Read the model definition and answer for the solid it produces. Units are mm, in the model's axes. Coordinates: 2 decimals unless noted, no trailing zeros. Write each loop counter-clockwise with the first axis right and the second up, starting at its lowest first coordinate (ties: lowest second). Pieces come first, ordered by that corner, then holes.
Item 1: Section C-C (z = -12) is taken. Give the vertices of the cut face in (x, y).
Item 2: Straight lines are drawn through the part: probe 1 along Z at (x, y) = (36, 1.5); probe 2 along X at (y, z) = (0.35, -63.94); probe 3 along X at (y, z) = (1.05, -17). For each, find the intervals that lie inside material, in ascending order.
Item 3: Section B-B (x = 6) is taken. Give the vertices of the cut face in (y, z).
Item 4: Section A-A (z = -48) is taken. Give the vertices of the cut face in (x, y).
Item 5: Each of these flat-tipped pins is pushed along its axis until it touches: P1, Ø2, axis at y = 1.5, z = -30.5, coming from the -X side; P2, Ø1.2, axis at y = -0.5, z = -38, coming from the +X side. Where does it stop, or does it pass through?
from build123d import *

# Parameters (mm, degrees)
SKETCH5_W           = 36.75
SKETCH5_H           = 66.29
BOSS_EXTRUDE3_DEPTH = 1
FILLET1_R           = 2
FILLET2_R           = 2
SKETCH7_R           = 1
CUT_EXTRUDE1_DEPTH  = 2
SKETCH9_W           = 4.683907435
SKETCH9_H           = 11.166934783
SKETCH9_W_2         = 3.743745131
SKETCH9_H_2         = 8.450578132
SKETCH9_W_3         = 2.561846092
SKETCH9_H_3         = 4.440718541
SKETCH9_H_4         = 4.716987875
SKETCH9_W_4         = 5.346352719
SKETCH9_H_5         = 7.570803243
BOSS_EXTRUDE5_DEPTH = 3
SKETCH11_W          = 2
SKETCH11_H          = 1.271998182
SKETCH11_H_2        = 1.351132692
BOSS_EXTRUDE6_DEPTH = 1
SKETCH12_W          = 2
SKETCH12_H          = 2
BOSS_EXTRUDE7_DEPTH = 2
SKETCH13_W          = 29.25
SKETCH13_H          = 59.29
BOSS_EXTRUDE8_DEPTH = 1.5


with BuildPart() as part:
    # Sketch5 → Boss-Extrude3 (new body)
    with BuildSketch(Plane(origin=(0, 0, 0), x_dir=(1, 0, 0), z_dir=(0, 1, 0))):
        with Locations((18.375, 33.145)):
            Rectangle(SKETCH5_W, SKETCH5_H)
    extrude(amount=BOSS_EXTRUDE3_DEPTH)

    # Fillet1
    fillet1_edges = [part.edges().sort_by_distance(p)[0] for p in [
        (0, 0.5, 0),
    ]]
    fillet(fillet1_edges, radius=FILLET1_R)

    # Fillet2
    fillet2_edges = [part.edges().sort_by_distance(p)[0] for p in [
        (0, 0.5, -66.29),
        (36.75, 0.5, -66.29),
        (36.75, 0.5, 0),
    ]]
    fillet(fillet2_edges, radius=FILLET2_R)

    # Sketch7 → Cut-Extrude1 (cut)
    with BuildSketch(Plane(origin=(0, 1, 0), x_dir=(1, 0, 0), z_dir=(0, 1, 0))):
        with Locations(Location((2.15, 63.94, 0), (0, 0, 270))):
            Circle(SKETCH7_R)
        with Locations(Location((34.5, 63.94, 0), (0, 0, 270))):
            Circle(SKETCH7_R)
        with Locations(Location((2.15, 2.52, 0), (0, 0, 270))):
            Circle(SKETCH7_R)
        with Locations(Location((34.5, 2.52, 0), (0, 0, 270))):
            Circle(SKETCH7_R)
    extrude(amount=-CUT_EXTRUDE1_DEPTH, mode=Mode.SUBTRACT)

    # Sketch9 → Boss-Extrude5 (add)
    with BuildSketch(Plane(origin=(0, 1, 0), x_dir=(1, 0, 0), z_dir=(0, 1, 0))):
        with Locations((2.341953718, 11.952713426)):
            Rectangle(SKETCH9_W, SKETCH9_H)
        with Locations((34.878127435, 23.466626346)):
            Rectangle(SKETCH9_W_2, SKETCH9_H_2)
        with Locations((35.469076954, 15.315821547)):
            Rectangle(SKETCH9_W_3, SKETCH9_H_3)
        with Locations((35.469076954, 8.727739972)):
            Rectangle(SKETCH9_W_3, SKETCH9_H_4)
        with Locations((2.67317636, 23.498188372)):
            Rectangle(SKETCH9_W_4, SKETCH9_H_5)
    extrude(amount=BOSS_EXTRUDE5_DEPTH)

    # Sketch11 → Boss-Extrude6 (add)
    with BuildSketch(Plane(origin=(36.75, 0, 0), x_dir=(0, 0, -1), z_dir=(1, 0, 0))):
        with Locations((8.727739971, 2.5)):
            Rectangle(SKETCH11_W, SKETCH11_H)
        with Locations((15.315821546, 2.5)):
            Rectangle(SKETCH11_W, SKETCH11_H_2)
    extrude(amount=BOSS_EXTRUDE6_DEPTH)

    # Sketch12 → Boss-Extrude7 (add)
    with BuildSketch(Plane(origin=(36.75, 0, 0), x_dir=(0, 0, -1), z_dir=(1, 0, 0))):
        with Locations((23.466626346, 2.5)):
            Rectangle(SKETCH12_W, SKETCH12_H)
    extrude(amount=BOSS_EXTRUDE7_DEPTH)

    # Sketch13 → Boss-Extrude8 (add)
    with BuildSketch(Plane.XZ):
        with Locations((18.625, -36.145)):
            Rectangle(SKETCH13_W, SKETCH13_H)
    extrude(amount=BOSS_EXTRUDE8_DEPTH)


solid = part.part
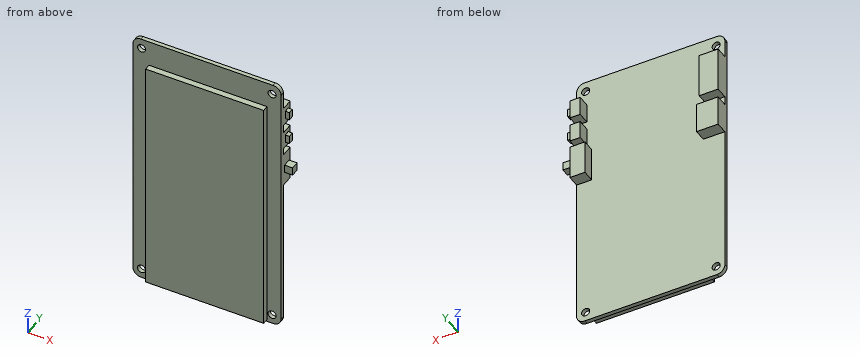
Established:
1. outline: (0, 0) - (4, 0) - (4, -1.5) - (33.25, -1.5) - (33.25, 0) - (36.75, 0) - (36.75, 1) - (4.68, 1) - (4.68, 4) - (0, 4) - close
2. probe 1: z = -27.69 to -19.24, -17.54 to -13.1, -11.09 to -6.37
2. probe 2: x = 0 to 1.15, 3.15 to 33.5, 35.5 to 36.75
2. probe 3: x = 0 to 4.68, 34.19 to 36.75
3. outline: (-1.5, -65.79) - (0, -65.79) - (0, -66.29) - (1, -66.29) - (1, 0) - (0, 0) - (0, -6.5) - (-1.5, -6.5) - close
4. outline: (0, 0) - (4, 0) - (4, -1.5) - (33.25, -1.5) - (33.25, 0) - (36.75, 0) - (36.75, 1) - (0, 1) - close
5. P1: stops at x = 0
5. P2: stops at x = 36.75
